For this review, take the finished solid that the model builds, in its own axes (mm). A direction names the side the tool comes from. Coordinates: 2 decimals unless noted, no trailing zeros. Write each loop counter-clockwise with the first axis right and the second up, starting at its lowest first coordinate (ties: lowest second). Pieces come first, ordered by that corner, then holes. Notation, with made-up numbers: (45.5, -16) - (69.5, -16) arc R14 ccw to (69.5, 2) - close; hole circle Ø3 at (-19, 85.5). An arc over 180 degrees is marked (long way). Use one line per item in the form item = value. Start each with the question number.
1) We need section D-D (y = -3). Give the boundary of the cut face in (x, z), plus the area to 3 significant figures.
2) Tool access review of faces 1 (the flat face through (0, 4.4, 12)), 2 (the flat face through (0, -4.4, 12)), 3 (the flat face through (-1, 0.7, 20)), 4 (the flat face through (0, -1.9, 20)): name each direction out of +Z, -Z, +X, -X, +Y, -Y from which nothing blocks a thin tool from reaching the whole face with its end or side.
3) We need section B-B (y = 0). Give the boundary of the cut face in (x, z).
4) For L1, parallel to Z at x = 1.75, y = 3.5; L2, parallel to X at y = -3, z = 2.5; L3, parallel to Y at x = 4, z = 11.5, list the stretches that pass through material, from the lowest coordinate up. Write a range as from..to.
5) We need section A-A (x = 0). Give the boundary of the cut face in (y, z), plus the area to 3 significant figures.
6) We need section C-C (z = 9.75). Give the boundary of the cut face in (x, y).
7) Insertion check: P1, Ø0.5, axis at x = 0, y = -4.5, coming from the -Z side; P2, Ø1.1, axis at x = 0.5, y = 4.5, coming from the -Z side; P3, Ø0.6, axis at x = 1.5, z = 20, coming from the +Y side; P4, Ø5, axis at y = -3, z = 14, coming from the +X side. Each pin has a flat end and moves straight along its axis. Give the tip position at first contact, or say it passes through.
```python
from build123d import *

# Parameters (mm, degrees)
F0_R     = 5
F1_DEPTH = 19
F3_DEPTH = 12
F4_W     = 1.4
F4_H     = 1.2
F4_W_2   = 1.2
F4_H_2   = 1.4
F5_DEPTH = 2


with BuildPart() as f1:
    # F0 (on Top) → F1 (new body)
    with BuildSketch(Plane.XY):
        Circle(F0_R)
    extrude(amount=F1_DEPTH)

    # F2 (on face) → F3 (cut)
    with BuildSketch(Plane(origin=(0, 0, 0), x_dir=(1, 0, 0), z_dir=(0, 0, -1))):
        with BuildLine():
            Line((-3, 4), (3, 4))
            ThreePointArc((3, 4), (0, 5), (-3, 4))
        make_face()
        with BuildLine():
            ThreePointArc((-3, -4), (0, -5), (3, -4))
            Line((3, -4), (-3, -4))
        make_face()
    extrude(amount=-F3_DEPTH, mode=Mode.SUBTRACT)

    # F4 (on face) → F5 (join)
    with BuildSketch(Plane.XY.offset(19)):
        with Locations((0, 1.3)):
            Rectangle(F4_W, F4_H)
        with Locations((-1.3, 0)):
            Rectangle(F4_W_2, F4_H_2)
        Rectangle(F4_W, F4_H_2)
        with Locations((0, -1.3)):
            Rectangle(F4_W, F4_H)
        with Locations((1.3, 0)):
            Rectangle(F4_W_2, F4_H_2)
    extrude(amount=F5_DEPTH)


solid = f1.part
```
Determined:
q1.outline = (-4, 0) - (4, 0) - (4, 19) - (-4, 19) - close
q1.area = 152 mm²
q2.face_1 = -Z, +X, -X, +Y
q2.face_2 = -Z, +X, -X, -Y
q2.face_3 = +Z, -X, +Y
q2.face_4 = +Z, +X, -X, -Y
q3.outline = (-5, 0) - (5, 0) - (5, 19) - (1.9, 19) - (1.9, 21) - (-1.9, 21) - (-1.9, 19) - (-5, 19) - close
q4.L1 = 0..19
q4.L2 = -4..4
q4.L3 = -3..3
q5.outline = (-5, 12) - (-4, 12) - (-4, 0) - (4, 0) - (4, 12) - (5, 12) - (5, 19) - (1.9, 19) - (1.9, 21) - (-1.9, 21) - (-1.9, 19) - (-5, 19) - close
q5.area = 174 mm²
q6.outline = (-3, -4) - (3, -4) arc R5 ccw to (3, 4) - (-3, 4) arc R5 ccw to start
q7.P1 = 12
q7.P2 = 0
q7.P3 = 0.7
q7.P4 = 4.97
